Can you work these out from the model? Positions are in its coordinate system, mm. A direction names the side the tool comes from. Coordinates: 2 decimals unless noted, no trailing zeros. Write each loop counter-clockwise with the first axis right and the second up, starting at its lowest first coordinate (ties: lowest second). Pieces come first, ordered by that corner, then holes.
```python
from build123d import *

# Parameters (mm, degrees)
F0_W     = 304.8
F0_H     = 142.2400027159
F1_DEPTH = 156.21
F2_T     = -17.78
F4_R     = 5


with BuildPart() as f1:
    # F0 (on Front) → F1 (new body)
    with BuildSketch(Plane.XZ):
        with Locations((-94.085527584, 5.834210664)):
            Rectangle(F0_W, F0_H)
    extrude(amount=F1_DEPTH)

    # F2
    f2_openings = [f1.faces().sort_by_distance(p)[0] for p in [
        (-94.085528, -78.105, 76.954212),
    ]]
    offset(amount=F2_T, openings=f2_openings)


with BuildPart() as f1_1:
    # F3: moved
    add(f1.part.moved(Location((0, 0, -77.978))))

    # F4
    f4_edges = [f1_1.edges().sort_by_distance(p)[0] for p in [
        (-94.085528, -156.21, -1.023788),
        (-246.485528, -78.105, -1.023788),
        (-94.085528, 0, -1.023788),
        (58.314472, -78.105, -1.023788),
        (40.534472, -78.105, -1.023788),
        (-94.085528, -138.43, -1.023788),
        (-94.085528, -17.78, -1.023788),
        (-228.705528, -78.105, -1.023788),
        (-246.485528, -156.21, -72.143789),
        (58.314472, -156.21, -72.143789),
        (-246.485528, 0, -72.143789),
        (58.314472, 0, -72.143789),
    ]]
    fillet(f4_edges, radius=F4_R)


solid = f1_1.part
```
1. If we section it at B-B, the plane y = -122.5: List the corners of the cut face in (x, z) for me, plus the area to 3 significant figures.
2. If we section it at A-A, the plane z = -68: List the corners of the cut face in (x, y) for me.
3. If we section it at C-C, the plane x = -26: List the corners of the cut face in (y, z) for me.
4. Which directions (+Z, -Z, +X, -X, +Y, -Y) give clear straight access to the entire face, cutting with the end or side of a thin tool? Please do faces 1 (the face through (-96, -138.43, -65)), 2 (the face through (58.314, -77, -76)).
5. If I drill on L1, parallel to Y at x = -47, z = -85; L2, parallel to X at y = -42.5, z = -104; L3, parallel to Z at x = -41, y = -59, over which ranges is the centre line in solid material (lowest first)?
6. I'm going to push a flat-ended pin straight in: P1, Ø1, axis at x = -56.5, y = -71, coming from the +Z side. Where does the tip first touch, or does it pass through?
7. We'd pull the mould along Y, two halves only. Please class faces 3 (the face through (-96, 0, -74)), 4 (the face through (-228.706, -77, -67)), 5 (the face through (-96, -77, -143.264)): released by +Y, released by -Y, zero draft, split by the parting line, or undercut.
Answers:
1. outline: (-246.49, -143.26) - (58.31, -143.26) - (58.31, -6.02) arc R5 ccw to (53.31, -1.02) - (45.53, -1.02) arc R5 ccw to (40.53, -6.02) - (40.53, -125.48) - (-228.71, -125.48) - (-228.71, -6.02) arc R5 ccw to (-233.71, -1.02) - (-241.49, -1.02) arc R5 ccw to (-246.49, -6.02) - close
1. area: 9,820 mm2
2. outline: (-246.49, -151.21) arc R5 ccw to (-241.49, -156.21) - (53.31, -156.21) arc R5 ccw to (58.31, -151.21) - (58.31, -5) arc R5 ccw to (53.31, 0) - (-241.49, 0) arc R5 ccw to (-246.49, -5) - close; hole (-228.71, -138.43) - (40.53, -138.43) - (40.53, -17.78) - (-228.71, -17.78) - close
3. outline: (-156.21, -143.26) - (0, -143.26) - (0, -6.02) arc R5 ccw to (-5, -1.02) - (-12.78, -1.02) arc R5 ccw to (-17.78, -6.02) - (-17.78, -125.48) - (-138.43, -125.48) - (-138.43, -6.02) arc R5 ccw to (-143.43, -1.02) - (-151.21, -1.02) arc R5 ccw to (-156.21, -6.02) - close
4. face 1: +Z
4. face 2: +Z, -Z, +X, +Y, -Y
5. L1: y = -156.21 to -138.43, -17.78 to 0
5. L2: x = -246.49 to -228.71, 40.53 to 58.31
5. L3: z = -143.26 to -125.48
6. P1: stops at z = -125.48
7. face 3: released by +Y
7. face 4: undercut
7. face 5: zero draft
